Build history of the part. All positions in model axes, mm. Face numbers are marked on the shaded views. A direction names the side the tool comes from. Give positions to 0.01 mm unless a question says otherwise; leave off trailing zeros. Order: outer loops, then holes, each group sorted by start corner. A loop starts at its lowest first (then second) coordinate and runs counter-clockwise, first axis right, second up. Notation, with made-up numbers: M -23,-9 L 3,-9 A22 ccw 3,22 Z; hole C 19.5,15.25 d9. An arc over 180 degrees is marked long. Use CSV: the item, a comma, the result in double quotes. Start each with the question number.
Item 1: Two-plate mould, pull along Y, no slides. Class the marked faces 1, 2, 3 and 4: pulls with the +Y half, pulls with the -Y half, needs draft (parallel to the pull), parting line crosses it, or undercut.
Item 2: Which spindle directions (+Z, -Z, +X, -X, +Y, -Y) get a long thin tool onto all of the face, cutting with end or side? Do the marked faces 5, 6 and 7. Say none if no direction does.
Item 3: Band-saw the part on C-C on x = 13. Write the cut outline in (y, z), plus the area to 3 significant figures.
Item 4: Pin check, flat tips, straight feed: P1, Ø5.5, axis at x = 0, y = 0, coming from the -Z side; P2, Ø2, axis at y = -10.5, z = 3, coming from the +X side; P3, Ø1, axis at x = -17.5, z = 3.5, coming from the +Y side; P4, Ø4, axis at x = 1, z = 3.5, coming from the -Y side. Stop position of each tip, or through.
Item 5: Band-saw the part on D-D on y = 0. Write the cut outline in (x, z), plus the area to 3 significant figures.
Item 6: Wall check: line 1 along Y through (x, z) = (-12, 2); line 2 along X through (y, z) = (-4, 1); line 3 along X through (y, z) = (-0.5, 3). Give the ranges that are in metal, low to high.
Item 7: Band-saw the part on A-A on y = 17. Write the cut outline in (x, z), plus the area to 3 significant figures.
Item 8: Band-saw the part on B-B on z = 1. Give the number of separate pieces and of enclosed holes in the cut face, plus the area to 3 significant figures.
from build123d import *

# Parameters (mm, degrees)
F0_R     = 3.5
F1_DEPTH = 7.8


# Not quite as in the source:
# - the program builds the solid bodies; features that only make, move or delete a surface that nothing else refers to are left out


with BuildPart() as f1:
    # F0 (on Top) → F1 (new body)
    with BuildSketch(Plane.XY):
        with BuildLine():
            ThreePointArc((16.5459263903, -18.417339772), (21.4411884767, -12.3790759388), (24.2228473078, -5.1205226972))
            Line((24.2228473078, -5.1205226972), (17.7308233658, 6.1239926144))
            Line((17.7308233658, 6.1239926144), (10.6070663534, 6.1239926144))
            Line((10.6070663534, 6.1239926144), (14.1689448596, 12.2933471575))
            Line((14.1689448596, 12.2933471575), (7.6769209175, 23.5378624692))
            ThreePointArc((7.6769209175, 23.5378624692), (0, 24.7581518775), (-7.6769209175, 23.5378624692))
            Line((-7.6769209175, 23.5378624692), (-14.1689448596, 12.2933471575))
            Line((-14.1689448596, 12.2933471575), (-10.6070663534, 6.1239926144))
            Line((-10.6070663534, 6.1239926144), (-17.7308233658, 6.1239926144))
            Line((-17.7308233658, 6.1239926144), (-24.2228473078, -5.1205226972))
            ThreePointArc((-24.2228473078, -5.1205226972), (-21.4411884767, -12.3790759388), (-16.5459263903, -18.417339772))
            Line((-16.5459263903, -18.417339772), (-3.5618785062, -18.417339772))
            Line((-3.5618785062, -18.417339772), (0, -12.2479852289))
            Line((0, -12.2479852289), (3.5618785062, -18.417339772))
            Line((3.5618785062, -18.417339772), (16.5459263903, -18.417339772))
        make_face()
        Polygon((-6.408587988, -14.9), (-16.1080725104, -14.9), (-20.9578147716, -6.5), (-16.1080725104, 1.9), (-6.408587988, 1.9), (-1.5588457268, -6.5), align=None, mode=Mode.SUBTRACT)
        Polygon((16.1080725104, 1.9), (20.9578147716, -6.5), (16.1080725104, -14.9), (6.408587988, -14.9), (1.5588457268, -6.5), (6.408587988, 1.9), align=None, mode=Mode.SUBTRACT)
        Circle(F0_R, mode=Mode.SUBTRACT)
        Polygon((9.6994845224, 13), (4.8497422612, 4.6), (-4.8497422612, 4.6), (-9.6994845224, 13), (-4.8497422612, 21.4), (4.8497422612, 21.4), align=None, mode=Mode.SUBTRACT)
    extrude(amount=F1_DEPTH)


solid = f1.part
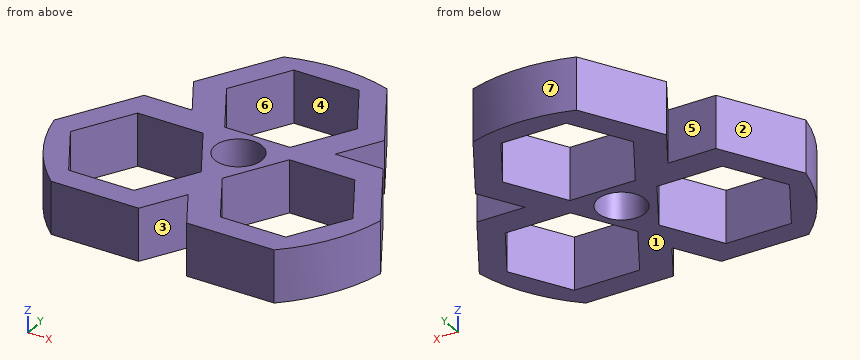
Model answer:
1,face 1,"needs draft"
1,face 2,"pulls with the +Y half"
1,face 3,"pulls with the -Y half"
1,face 4,"undercut"
2,face 5,"+Z, -Z, -X"
2,face 6,"+Z, -Z"
2,face 7,"+Z, -Z, +Y"
3,outline,"M -18.42,0 L -14.9,0 L -14.9,7.8 L -18.42,7.8 Z; M 1.9,0 L 6.12,0 L 6.12,7.8 L 1.9,7.8 Z; M 10.27,0 L 14.32,0 L 14.32,7.8 L 10.27,7.8 Z"
3,area,"92.0 mm^2"
4,P1,"passes through"
4,P2,"stops at x = 22.86"
4,P3,"stops at y = 6.12"
4,P4,"stops at y = -17.44"
5,outline,"M -21.27,0 L -17.21,0 L -17.21,7.8 L -21.27,7.8 Z; M -5.31,0 L -3.5,0 L -3.5,7.8 L -5.31,7.8 Z; M 3.5,0 L 5.31,0 L 5.31,7.8 L 3.5,7.8 Z; M 17.21,0 L 21.27,0 L 21.27,7.8 L 17.21,7.8 Z"
5,area,"91.6 mm^2"
6,line 1,"y = -18.42 to -14.9, 1.9 to 6.12, 8.54 to 16.05"
6,line 2,"x = -23.58 to -19.51, -3 to 3, 19.51 to 23.58"
6,line 3,"x = -21.56 to -17.49, -5.02 to -3.46, 3.46 to 5.02, 17.49 to 21.56"
7,outline,"M -11.45,0 L -7.39,0 L -7.39,7.8 L -11.45,7.8 Z; M 7.39,0 L 11.45,0 L 11.45,7.8 L 7.39,7.8 Z"
7,area,"63.4 mm^2"
8,separate pieces,"1"
8,enclosed holes,"4"
8,area,"656 mm^2"
